from build123d import *

# Parameters (mm, degrees)
SKETCH_1_W          = 88
SKETCH_1_H          = 70
EXTRUDE_1_DEPTH     = 35
SKETCH_3_W          = 88
SKETCH_3_H          = 50
EXTRUDE_2_DEPTH     = 30
SKETCH_6_R          = 13.5
EXTRUDE_3_DEPTH     = 3
EXTRUDE_4_DEPTH     = 5
CUT_EXTRUDE_1_REACH = 95.963
SKETCH_8_R          = 1.5


with BuildPart() as part:
    # 草图1 → 凸台-拉伸1 (new body)
    with BuildSketch(Plane.XY):
        Rectangle(SKETCH_1_W, SKETCH_1_H)
    extrude(amount=EXTRUDE_1_DEPTH)

    # 草图3 → 凸台-拉伸2 (add)
    with BuildSketch(Plane(origin=(0, 0, 0), x_dir=(-1, 0, 0), z_dir=(0, 0, -1))):
        with Locations((0, 10)):
            Rectangle(SKETCH_3_W, SKETCH_3_H)
    extrude(amount=EXTRUDE_2_DEPTH)

    # 草图6 → 凸台-拉伸3 (add)
    with BuildSketch(Plane(origin=(44, 0, 0), x_dir=(0, 0, -1), z_dir=(1, 0, 0))):
        with Locations(Location((-18, 0, 0), (0, 0, 180))):
            Circle(SKETCH_6_R)
    extrude(amount=EXTRUDE_3_DEPTH)

    # 草图7 → 凸台-拉伸4 (add)
    with BuildSketch(Plane(origin=(47, 0, 0), x_dir=(0, 0, -1), z_dir=(1, 0, 0))):
        with BuildLine():
            Line((-16.042793618, 0), (-16.042793618, -18.740555958))
            ThreePointArc((-16.042793618, -18.740555958), (-18, -20.697762339), (-19.957206382, -18.740555958))
            Line((-19.957206382, -18.740555958), (-19.957206382, 0))
            ThreePointArc((-19.957206382, 0), (-18, 1.957206382), (-16.042793618, 0))
        make_face()
    extrude(amount=EXTRUDE_4_DEPTH)

    # 草图8 → 切除-拉伸1 (cut, up to next)
    with BuildSketch(Plane(origin=(0, 35, 0), x_dir=(1, 0, 0), z_dir=(0, 1, 0)), mode=Mode.PRIVATE) as cut_extrude_1_sk1:
        with Locations(Location((-22, 19, 0), (0, 0, 270))):
            Circle(SKETCH_8_R)
    cut_extrude_1_tool1 = extrude(cut_extrude_1_sk1.sketch, amount=-CUT_EXTRUDE_1_REACH, mode=Mode.PRIVATE) & part.part
    # 草图8 → 切除-拉伸1 (cut, up to next)
    with BuildSketch(Plane(origin=(0, 35, 0), x_dir=(1, 0, 0), z_dir=(0, 1, 0)), mode=Mode.PRIVATE) as cut_extrude_1_sk2:
        with Locations(Location((-2, 19, 0), (0, 0, 270))):
            Circle(SKETCH_8_R)
    cut_extrude_1_tool2 = extrude(cut_extrude_1_sk2.sketch, amount=-CUT_EXTRUDE_1_REACH, mode=Mode.PRIVATE) & part.part
    add(cut_extrude_1_tool1.solids().sort_by_distance((-22, 35, -19))[0], mode=Mode.SUBTRACT)
    add(cut_extrude_1_tool2.solids().sort_by_distance((-2, 35, -19))[0], mode=Mode.SUBTRACT)


solid = part.part
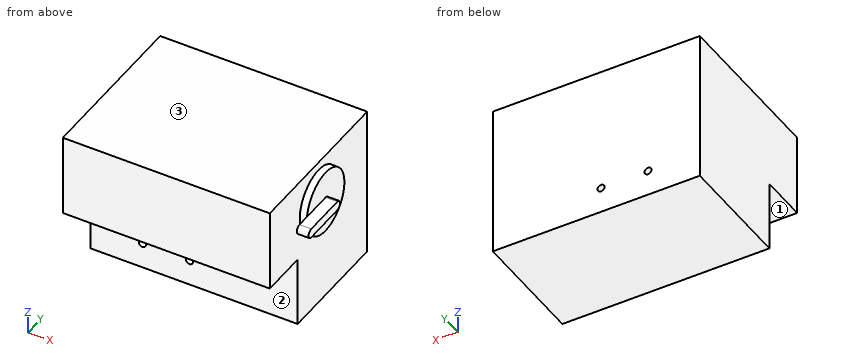
For this review, take the finished solid that the model builds, in its own axes (mm). Face numbers are marked on the shaded views. Coordinates: 2 decimals unless noted, no trailing zeros. Order: outer loops, then holes, each group sorted by start corner. A loop starts at its lowest first (then second) coordinate and runs counter-clockwise, first axis right, second up. Notation, with made-up numbers: (49.25, 63) -> (63.25, 63) arc R16 cw to (63.25, 77) -> close; hole circle Ø9 at (23.25, 20). An arc over 180 degrees is marked (long way). Return JSON: item names as keys, results as strings.
1. We need section A-A on x = -22. Write out the cut boundary in (y, z).
Answer block:
{"outline": "(-35, 0) -> (-15, 0) -> (-15, -17.5) -> (35, -17.5) -> (35, 35) -> (-35, 35) -> close; (-15, -30) -> (35, -30) -> (35, -20.5) -> (-15, -20.5) -> close"}
2. For pin 1 Ø4 at (x, z) = (-22, -19) entering from -Y; pin 2 Ø5.5 at (x, y) = (50, -6) entering from +Z; pin 3 Ø2.5 at (x, z) = (-2, -19) entering from +Y; pin 4 Ø12 at (y, z) = (-17.5, -14) entering from +X, all flat-tipped, find the tip position at first contact; note any pin that passes through.
Answer block:
{"pin 1": "y = -15", "pin 2": "z = 19.96", "pin 3": "through", "pin 4": "x = 44"}
3. We need section C-C on z = 18. Write out the cut boundary in (x, y), and give its area (3 significant figures).
Answer block:
{"outline": "(-44, -35) -> (44, -35) -> (44, -13.5) -> (47, -13.5) -> (47, -20.7) -> (52, -20.7) -> (52, 1.96) -> (47, 1.96) -> (47, 13.5) -> (44, 13.5) -> (44, 35) -> (-44, 35) -> close", "area": "6,350 mm²"}
4. The part is to be moulded in two halves that separate along Z. For the marked faces 1, 2 and 3, say which applies: +Z half, -Z half, draft (parallel to the pull), parting line (faces both ways), or undercut.
Answer block:
{"face 1": "-Z half", "face 2": "draft", "face 3": "+Z half"}
5. We need section D-D on x = 12. Write out the cut boundary in (y, z).
Answer block:
{"outline": "(-35, 0) -> (-15, 0) -> (-15, -30) -> (35, -30) -> (35, 35) -> (-35, 35) -> close"}
6. For line 1 (X direction, y = 2, z = -19); line 2 (X direction, y = -10.5, z = -11.5); line 3 (Y direction, x = -15, z = -9.5), list the stretches that pass through material, from the lowest coordinate up. Write a range as from..to.
Answer block:
{"line 1": "-44..-23.5, -20.5..-3.5, -0.5..44", "line 2": "-44..44", "line 3": "-15..35"}
7. We need section B-B on y = 6. Write out the cut boundary in (x, z), and give its area (3 significant figures).
Answer block:
{"outline": "(-44, -30) -> (44, -30) -> (44, 5.91) -> (47, 5.91) -> (47, 30.09) -> (44, 30.09) -> (44, 35) -> (-44, 35) -> close; hole circle Ø3 at (-22, -19); hole circle Ø3 at (-2, -19)", "area": "5,780 mm²"}
